from build123d import *

# Parameters (mm, degrees)
SKETCH1_W               = 19.05
SKETCH1_H               = 50.8
BOSS_EXTRUDE1_DEPTH     = 1.5875
F_1_4_CLEARANCE_HOLE1_D = 6.5278
FILLET1_R               = 6.35


with BuildPart() as part:
    # Sketch1 → Boss-Extrude1 (new, symmetric)
    with BuildSketch(Plane(origin=(0, 0, 0), x_dir=(0, 0, -1), z_dir=(1, 0, 0))):
        Rectangle(SKETCH1_W, SKETCH1_H)
    extrude(amount=BOSS_EXTRUDE1_DEPTH, both=True)

    # 1/4 Clearance Hole1 (through all)
    with Locations(Plane(origin=(1.5875, 0, 0), x_dir=(0, 0, -1), z_dir=(1, 0, 0))):
        with Locations((0, 12.7), (0, -12.7)):
            Hole(F_1_4_CLEARANCE_HOLE1_D / 2)

    # Fillet1
    fillet1_edges = [part.edges().sort_by_distance(p)[0] for p in [
        (0, -25.4, -9.525),
        (0, -25.4, 9.525),
        (0, 25.4, 9.525),
        (0, 25.4, -9.525),
    ]]
    fillet(fillet1_edges, radius=FILLET1_R)


solid = part.part
Input: part model. Units: mm. Frame: model coordinates. Round coordinates to 2 decimals unless told otherwise and drop trailing zeros. Order: outer loops, then holes, each group sorted by start corner. A loop starts at its lowest first (then second) coordinate and runs counter-clockwise, first axis right, second up.
1. Cut plane A-A, the plane z = 0. Output: boundary loops of the cut face in (x, y), then the cut area to 3 significant figures.
The answers:
outline: (-1.59, -25.4) - (1.59, -25.4) - (1.59, -15.96) - (-1.59, -15.96) - close; (-1.59, -9.44) - (1.59, -9.44) - (1.59, 9.44) - (-1.59, 9.44) - close; (-1.59, 15.96) - (1.59, 15.96) - (1.59, 25.4) - (-1.59, 25.4) - close
area: 120 mm2
2. Cut plane D-D, the plane z = -5.75. Output: boundary loops of the cut face in (x, y), then the cut area to 3 significant figures.
The answers:
outline: (-1.59, -24.85) - (1.59, -24.85) - (1.59, 24.85) - (-1.59, 24.85) - close
area: 158 mm2
3. Mould query, pull axis Z, two halves, no side actions, for faces 1 (the face through (-1.588, 0, 0)), 2 (the face through (0, 0, 9.525)), 3 (the face through (-0.022, -9.464, -0.425)). Classes: released by +Z, released by -Z, zero draft, split by the parting line, or undercut.
The answers:
face 1: zero draft
face 2: released by +Z
face 3: undercut
4. Material intervals for line 1 (Y direction, x = 0.7, z = 0); line 2 (Z direction, x = 0.2, y = 12.5) (3 decimals); line 3 (Y direction, x = 0.3, z = 1.75), sorted ascending.
The answers:
line 1: y = -25.4 to -15.96, -9.44 to 9.44, 15.96 to 25.4
line 2: z = -9.525 to -3.258, 3.258 to 9.525
line 3: y = -25.4 to -15.46, -9.94 to 9.94, 15.46 to 25.4
5. Cut plane C-C, the plane y = 12.7. Output: boundary loops of the cut face in (x, z) (1 decimal), then the cut area to 3 significant figures.
The answers:
outline: (-1.6, -9.5) - (1.6, -9.5) - (1.6, -3.3) - (-1.6, -3.3) - close; (-1.6, 3.3) - (1.6, 3.3) - (1.6, 9.5) - (-1.6, 9.5) - close
area: 39.8 mm2
6. Cut plane B-B, the plane x = -0.4. Output: boundary loops of the cut face in (y, z) (3 decimals).
The answers:
outline: (-25.4, -3.175) arc R6.35 ccw to (-19.05, -9.525) - (19.05, -9.525) arc R6.35 ccw to (25.4, -3.175) - (25.4, 3.175) arc R6.35 ccw to (19.05, 9.525) - (-19.05, 9.525) arc R6.35 ccw to (-25.4, 3.175) - close; hole circle Ø6.528 at (-12.7, 0); hole circle Ø6.528 at (12.7, 0)
